Source: CAD feature listing. Evaluate the final solid. Frame: model axes, mm. Face numbers are marked on the shaded views. A direction names the side the tool comes from. Give positions to 0.01 mm unless a question says otherwise; leave off trailing zeros. Loops run counter-clockwise (first coordinate to the right, second up) from the corner with the lowest first, then second, coordinate; pieces in that order, holes last. Notation, with made-up numbers: (27, 26) -> (57, 26) arc R19 cw to (57, 60) -> close; hole circle Ø2 at (5.5, 80). An arc over 180 degrees is marked (long way). Put each result on its own line as item: value.
```python
from build123d import *

# Parameters (mm, degrees)
SKETCH1_W                    = 96
SKETCH1_H                    = 1
BASE_FLANGE1_DEPTH           = 329.72
EDGE_FLANGE1_STRIP_W         = 5.4732
EDGE_FLANGE1_STRIP_H         = 1
EDGE_FLANGE1_STRIP_CUT_DEPTH = 96
EDGE_FLANGE1_DEPTH           = 96
EDGE_FLANGE2_STRIP_W         = 5.4732
EDGE_FLANGE2_STRIP_H         = 1
EDGE_FLANGE2_STRIP_CUT_DEPTH = 96
EDGE_FLANGE2_DEPTH           = 96
EDGE_FLANGE3_STRIP_W         = 5.4732
EDGE_FLANGE3_STRIP_H         = 1
EDGE_FLANGE3_STRIP_CUT_DEPTH = 96
EDGE_FLANGE3_DEPTH           = 96
EDGE_FLANGE4_STRIP_W         = 5.4732
EDGE_FLANGE4_STRIP_H         = 1
EDGE_FLANGE4_STRIP_CUT_DEPTH = 96
EDGE_FLANGE4_DEPTH           = 96
CUT_EXTRUDE1_DEPTH           = 10


# Sheet-metal steps are written as plain solids
with BuildPart() as part:
    # Sketch1 → Base-Flange1 (new body)
    with BuildSketch(Plane.XY):
        with Locations((48, -0.5)):
            Rectangle(SKETCH1_W, SKETCH1_H)
    extrude(amount=BASE_FLANGE1_DEPTH)

    # Edge-Flange1 strip (across the edge) → Edge-Flange1 strip cut (cut)
    with BuildSketch(Plane(origin=(0, 0, 329.72), x_dir=(0, 0, -1), z_dir=(1, 0, 0))):
        with Locations((-1, -0.5)):
            Rectangle(EDGE_FLANGE1_STRIP_W, EDGE_FLANGE1_STRIP_H)
    extrude(amount=EDGE_FLANGE1_STRIP_CUT_DEPTH, mode=Mode.SUBTRACT)

    # Edge-Flange1 section (across the edge) → Edge-Flange1 (add)
    with BuildSketch(Plane(origin=(0, 0, 329.72), x_dir=(0, 0, -1), z_dir=(1, 0, 0))):
        with BuildLine():
            Line((0, 0.7366), (0, 35))
            Line((0, 35), (1, 35))
            Line((1, 35), (1, 0.7366))
            ThreePointArc((1, 0.7366), (1.215745145, 0.215745145), (1.7366, 0))
            Line((1.7366, 0), (1.7366, -1))
            ThreePointArc((1.7366, -1), (0.508638364, -0.491361636), (0, 0.7366))
        make_face()
    extrude(amount=EDGE_FLANGE1_DEPTH)

    # Edge-Flange2 strip (across the edge) → Edge-Flange2 strip cut (cut)
    with BuildSketch(Plane.ZY.offset(-96)):
        with Locations((-1, -0.5)):
            Rectangle(EDGE_FLANGE2_STRIP_W, EDGE_FLANGE2_STRIP_H)
    extrude(amount=EDGE_FLANGE2_STRIP_CUT_DEPTH, mode=Mode.SUBTRACT)

    # Edge-Flange2 section (across the edge) → Edge-Flange2 (add)
    with BuildSketch(Plane.ZY.offset(-96)):
        with BuildLine():
            Line((0, 0.7366), (0, 35))
            Line((0, 35), (1, 35))
            Line((1, 35), (1, 0.7366))
            ThreePointArc((1, 0.7366), (1.215745145, 0.215745145), (1.7366, 0))
            Line((1.7366, 0), (1.7366, -1))
            ThreePointArc((1.7366, -1), (0.508638364, -0.491361636), (0, 0.7366))
        make_face()
    extrude(amount=EDGE_FLANGE2_DEPTH)

    # Edge-Flange3 strip (across the edge) → Edge-Flange3 strip cut (cut)
    with BuildSketch(Plane(origin=(0, 35, 328.72), x_dir=(0, -1, 0), z_dir=(1, 0, 0))):
        with Locations((-1, -0.5)):
            Rectangle(EDGE_FLANGE3_STRIP_W, EDGE_FLANGE3_STRIP_H)
    extrude(amount=EDGE_FLANGE3_STRIP_CUT_DEPTH, mode=Mode.SUBTRACT)

    # Edge-Flange3 section (across the edge) → Edge-Flange3 (add)
    with BuildSketch(Plane(origin=(0, 35, 328.72), x_dir=(0, -1, 0), z_dir=(1, 0, 0))):
        with BuildLine():
            Line((0, 0.7366), (0, 27))
            Line((0, 27), (1, 27))
            Line((1, 27), (1, 0.7366))
            ThreePointArc((1, 0.7366), (1.215745145, 0.215745145), (1.7366, 0))
            Line((1.7366, 0), (1.7366, -1))
            ThreePointArc((1.7366, -1), (0.508638364, -0.491361636), (0, 0.7366))
        make_face()
    extrude(amount=EDGE_FLANGE3_DEPTH)

    # Edge-Flange4 strip (across the edge) → Edge-Flange4 strip cut (cut)
    with BuildSketch(Plane(origin=(96, 35, 1), x_dir=(0, -1, 0), z_dir=(-1, 0, 0))):
        with Locations((-1, -0.5)):
            Rectangle(EDGE_FLANGE4_STRIP_W, EDGE_FLANGE4_STRIP_H)
    extrude(amount=EDGE_FLANGE4_STRIP_CUT_DEPTH, mode=Mode.SUBTRACT)

    # Edge-Flange4 section (across the edge) → Edge-Flange4 (add)
    with BuildSketch(Plane(origin=(96, 35, 1), x_dir=(0, -1, 0), z_dir=(-1, 0, 0))):
        with BuildLine():
            Line((0, 0.7366), (0, 27))
            Line((0, 27), (1, 27))
            Line((1, 27), (1, 0.7366))
            ThreePointArc((1, 0.7366), (1.215745145, 0.215745145), (1.7366, 0))
            Line((1.7366, 0), (1.7366, -1))
            ThreePointArc((1.7366, -1), (0.508638364, -0.491361636), (0, 0.7366))
        make_face()
    extrude(amount=EDGE_FLANGE4_DEPTH)

    # Sketch22 → Cut-Extrude1 (cut)
    with BuildSketch(Plane(origin=(0, 0, 0), x_dir=(1, 0, 0), z_dir=(0, 1, 0))):
        with BuildLine():
            Line((26, -214.9834), (26, -287.9834))
            ThreePointArc((26, -287.9834), (19, -294.9834), (12, -287.9834))
            Line((12, -287.9834), (12, -214.9834))
            ThreePointArc((12, -214.9834), (19, -207.9834), (26, -214.9834))
        make_face()
        with BuildLine():
            Line((26, -114.7366), (26, -41.7366))
            ThreePointArc((26, -41.7366), (19, -34.7366), (12, -41.7366))
            Line((12, -41.7366), (12, -114.7366))
            ThreePointArc((12, -114.7366), (19, -121.7366), (26, -114.7366))
        make_face()
    extrude(amount=-CUT_EXTRUDE1_DEPTH, mode=Mode.SUBTRACT)


solid = part.part
```
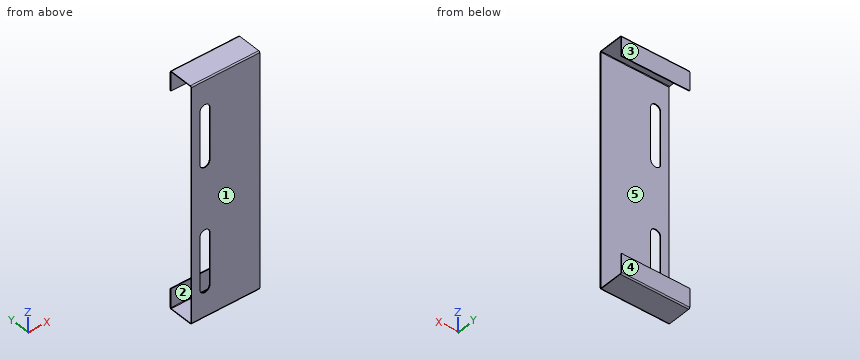
(1) Reachability of the marked faces 4 and 5 from +Z, -Z, +X, -X, +Y, -Y: full face, straight path, thin tool, end or side. Return the list, or none.
Calculated:
face 4: +Z, -Z, +X, -X, +Y
face 5: +X, -X
(2) Section C-C on z = 54. Return loops of the section in (x, y), then the cut area to 3 significant figures.
Calculated:
outline: (0, -1) -> (12, -1) -> (12, 0) -> (0, 0) -> close; (26, -1) -> (96, -1) -> (96, 0) -> (26, 0) -> close
area: 82.0 mm²
(3) Section B-B on y = 15.5. Return loops of the section in (x, z).
Calculated:
outline: (0, 0) -> (96, 0) -> (96, 1) -> (0, 1) -> close; (0, 328.72) -> (96, 328.72) -> (96, 329.72) -> (0, 329.72) -> close
(4) Draft query along Y for the marked faces 1, 2 and 3. Return one class per face: released by +Y, released by -Y, zero draft, split by the parting line, or undercut.
Calculated:
face 1: released by -Y
face 2: undercut
face 3: released by +Y
(5) Line query: probe 1 along Z at (x, y) = (16, 17); probe 2 along Y at (x, z) = (91.5, 315.5); probe 3 along Y at (x, z) = (78, 276). Output: solid intervals per line, ascending. Write a range as from..to.
Calculated:
probe 1: z = 0..1, 328.72..329.72
probe 2: y = -1..0, 34..35
probe 3: y = -1..0
(6) Section A-A on x = 19. Return loops of the section in (y, z).
Calculated:
outline: (-1, 1.74) arc R1.74 ccw to (0.74, 0) -> (33.26, 0) arc R1.74 ccw to (35, 1.74) -> (35, 28) -> (34, 28) -> (34, 1.74) arc R0.74 cw to (33.26, 1) -> (0.74, 1) arc R0.74 cw to (0, 1.74) -> (0, 34.74) -> (-1, 34.74) -> close; (-1, 121.74) -> (0, 121.74) -> (0, 207.98) -> (-1, 207.98) -> close; (-1, 294.98) -> (0, 294.98) -> (0, 327.98) arc R0.74 cw to (0.74, 328.72) -> (33.26, 328.72) arc R0.74 cw to (34, 327.98) -> (34, 301.72) -> (35, 301.72) -> (35, 327.98) arc R1.74 ccw to (33.26, 329.72) -> (0.74, 329.72) arc R1.74 ccw to (-1, 327.98) -> close
(7) First-contact query: P1, Ø0.8, axis at x = 34.5, y = 34.5, coming from the -Z side; P2, Ø1, axis at x = 56.5, z = 69.5, coming from the +Y side; P3, Ø1.1, axis at x = 63.5, y = 34.5, coming from the +Z side. Flat tips, straight axial feed; report the tip coordinate or a pass-through.
Calculated:
P1: stops at z = 0.21
P2: stops at y = 0
P3: stops at z = 329.58
